Verification items for the finished model (mm, model axes). A direction names the side the tool comes from. Give positions to 0.01 mm unless a question says otherwise; leave off trailing zeros.
from build123d import *

# Parameters (mm, degrees)
BOSS_EXTRUDE1_START = -13.97
BOSS_EXTRUDE1_DEPTH = 7.62
SKETCH3_W           = 157.48
SKETCH3_H           = 157.48
CUT_EXTRUDE1_DEPTH  = 1
SKETCH3_3_R         = 1.8
BOSS_EXTRUDE2_DEPTH = 37
FILLET1_R           = 1
SKETCH11_R          = 5.1
CUT_EXTRUDE2_DEPTH  = 12.7
SKETCH10_R          = 5
BOSS_EXTRUDE3_DEPTH = 12.5
FILLET2_R           = 1


# Read off the part's stored shape, not the designer's step: Boss-Extrude1
with BuildPart() as part:
    # Sketch1 → Revolve1 (revolve)
    with BuildSketch(Plane.YZ, mode=Mode.PRIVATE) as revolve1_sk:
        Polygon((0, 0), (-152.4, 0), (-152.4, -6.35), (-150.8, -6.35), (-150.8, -13.97), (-152.4, -13.97), (-152.4, -17.97), (-88.9, -17.97), (-88.9, -23.97), (-111.6, -30.32), (0, -30.32), align=None)
    revolve(revolve1_sk.sketch.rotate(Axis((0, 0, -30.32), (0, 0, 1)), 180), axis=Axis((0, 0, -30.32), (0, 0, 1)))

    # Boss-Extrude1 outline → Boss-Extrude1 (add)
    with BuildSketch(Plane.XY.offset(BOSS_EXTRUDE1_START)):
        with BuildLine():
            Line((150.751862012, 3.81), (152.352367556, 3.81))
            ThreePointArc((152.352367556, 3.81), (149.471676733, 29.731765076), (142.213257992, 54.782745927))
            Line((142.213257992, 54.782745927), (140.734583678, 54.170258971))
            ThreePointArc((140.734583678, 54.170258971), (147.902420285, 29.41962056), (150.751862012, 3.81))
        make_face()
        with BuildLine():
            ThreePointArc((142.213257992, -54.782745926), (149.471676733, -29.731765075), (152.352367556, -3.81))
            Line((152.352367556, -3.81), (150.751862012, -3.81))
            ThreePointArc((150.751862012, -3.81), (147.902420285, -29.41962056), (140.734583678, -54.170258971))
            Line((140.734583678, -54.170258971), (142.213257992, -54.782745926))
        make_face()
        with BuildLine():
            Line((137.818535923, 61.210221009), (139.297210238, 61.822707964))
            ThreePointArc((139.297210238, 61.822707964), (126.715968915, 84.668903512), (110.423469065, 105.035315393))
            Line((110.423469065, 105.035315393), (109.291740741, 103.903587069))
            ThreePointArc((109.291740741, 103.903587069), (125.385617535, 83.77999114), (137.818535923, 61.210221009))
        make_face()
        with BuildLine():
            ThreePointArc((110.423469065, -105.035315392), (126.715968915, -84.668903512), (139.297210238, -61.822707964))
            Line((139.297210238, -61.822707964), (137.818535923, -61.210221009))
            ThreePointArc((137.818535923, -61.210221009), (125.385617535, -83.77999114), (109.291740741, -103.903587069))
            Line((109.291740741, -103.903587069), (110.423469065, -105.035315392))
        make_face()
        with BuildLine():
            Line((103.903587069, 109.291740741), (105.035315393, 110.423469065))
            ThreePointArc((105.035315393, 110.423469065), (84.668903512, 126.715968915), (61.822707964, 139.297210238))
            Line((61.822707964, 139.297210238), (61.210221009, 137.818535923))
            ThreePointArc((61.210221009, 137.818535923), (83.77999114, 125.385617535), (103.903587069, 109.291740741))
        make_face()
        with BuildLine():
            ThreePointArc((61.822707964, -139.297210238), (84.668903512, -126.715968915), (105.035315393, -110.423469065))
            Line((105.035315393, -110.423469065), (103.903587069, -109.291740741))
            ThreePointArc((103.903587069, -109.291740741), (83.77999114, -125.385617535), (61.210221009, -137.818535923))
            Line((61.210221009, -137.818535923), (61.822707964, -139.297210238))
        make_face()
        with BuildLine():
            Line((54.170258971, 140.734583678), (54.782745927, 142.213257992))
            ThreePointArc((54.782745927, 142.213257992), (29.731765076, 149.471676733), (3.81, 152.352367556))
            Line((3.81, 152.352367556), (3.81, 150.751862012))
            ThreePointArc((3.81, 150.751862012), (29.41962056, 147.902420285), (54.170258971, 140.734583678))
        make_face()
        with BuildLine():
            ThreePointArc((3.81, -152.352367556), (29.731765076, -149.471676733), (54.782745927, -142.213257992))
            Line((54.782745927, -142.213257992), (54.170258971, -140.734583678))
            ThreePointArc((54.170258971, -140.734583678), (29.41962056, -147.902420285), (3.81, -150.751862012))
            Line((3.81, -150.751862012), (3.81, -152.352367556))
        make_face()
        with BuildLine():
            Line((-3.81, 150.751862012), (-3.81, 152.352367556))
            ThreePointArc((-3.81, 152.352367556), (-29.731765076, 149.471676733), (-54.782745927, 142.213257992))
            Line((-54.782745927, 142.213257992), (-54.170258971, 140.734583678))
            ThreePointArc((-54.170258971, 140.734583678), (-29.41962056, 147.902420285), (-3.81, 150.751862012))
        make_face()
        with BuildLine():
            ThreePointArc((-54.782745926, -142.213257992), (-29.731765075, -149.471676733), (-3.81, -152.352367556))
            Line((-3.81, -152.352367556), (-3.81, -150.751862012))
            ThreePointArc((-3.81, -150.751862012), (-29.41962056, -147.902420285), (-54.170258971, -140.734583678))
            Line((-54.170258971, -140.734583678), (-54.782745926, -142.213257992))
        make_face()
        with BuildLine():
            Line((-61.210221009, 137.818535923), (-61.822707964, 139.297210238))
            ThreePointArc((-61.822707964, 139.297210238), (-84.668903512, 126.715968915), (-105.035315393, 110.423469065))
            Line((-105.035315393, 110.423469065), (-103.903587069, 109.291740741))
            ThreePointArc((-103.903587069, 109.291740741), (-83.77999114, 125.385617535), (-61.210221009, 137.818535923))
        make_face()
        with BuildLine():
            ThreePointArc((-105.035315392, -110.423469065), (-84.668903512, -126.715968915), (-61.822707964, -139.297210238))
            Line((-61.822707964, -139.297210238), (-61.210221009, -137.818535923))
            ThreePointArc((-61.210221009, -137.818535923), (-83.77999114, -125.385617535), (-103.903587069, -109.291740741))
            Line((-103.903587069, -109.291740741), (-105.035315392, -110.423469065))
        make_face()
        with BuildLine():
            Line((-109.291740741, 103.903587069), (-110.423469065, 105.035315393))
            ThreePointArc((-110.423469065, 105.035315393), (-126.715968915, 84.668903512), (-139.297210238, 61.822707964))
            Line((-139.297210238, 61.822707964), (-137.818535923, 61.210221009))
            ThreePointArc((-137.818535923, 61.210221009), (-125.385617535, 83.77999114), (-109.291740741, 103.903587069))
        make_face()
        with BuildLine():
            ThreePointArc((-139.297210238, -61.822707964), (-126.715968915, -84.668903512), (-110.423469065, -105.035315393))
            Line((-110.423469065, -105.035315393), (-109.291740741, -103.903587069))
            ThreePointArc((-109.291740741, -103.903587069), (-125.385617535, -83.77999114), (-137.818535923, -61.210221009))
            Line((-137.818535923, -61.210221009), (-139.297210238, -61.822707964))
        make_face()
        with BuildLine():
            Line((-140.734583678, 54.170258971), (-142.213257992, 54.782745926))
            ThreePointArc((-142.213257992, 54.782745926), (-149.471676733, 29.731765075), (-152.352367556, 3.81))
            Line((-152.352367556, 3.81), (-150.751862012, 3.81))
            ThreePointArc((-150.751862012, 3.81), (-147.902420285, 29.41962056), (-140.734583678, 54.170258971))
        make_face()
        with BuildLine():
            ThreePointArc((-152.352367556, -3.81), (-149.471676733, -29.731765076), (-142.213257992, -54.782745927))
            Line((-142.213257992, -54.782745927), (-140.734583678, -54.170258971))
            ThreePointArc((-140.734583678, -54.170258971), (-147.902420285, -29.41962056), (-150.751862012, -3.81))
            Line((-150.751862012, -3.81), (-152.352367556, -3.81))
        make_face()
    extrude(amount=BOSS_EXTRUDE1_DEPTH)

    # Sketch3 → Cut-Extrude1 (cut)
    with BuildSketch(Plane(origin=(0, 0, -30.32), x_dir=(1, 0, 0), z_dir=(0, 0, -1))):
        Rectangle(SKETCH3_W, SKETCH3_H)
    extrude(amount=-CUT_EXTRUDE1_DEPTH, mode=Mode.SUBTRACT)

    # Sketch3<3> → Boss-Extrude2 (add)
    with BuildSketch(Plane(origin=(0, 0, -30.32), x_dir=(1, 0, 0), z_dir=(0, 0, -1))):
        with Locations(Location((0, 0, 0), (0, 0, 180))):
            Circle(SKETCH3_3_R)
    extrude(amount=-BOSS_EXTRUDE2_DEPTH)

    # Fillet1
    fillet1_edges = [part.edges().sort_by_distance(p)[0] for p in [
        (1.8, 0, 6.68),
    ]]
    fillet(fillet1_edges, radius=FILLET1_R)

    # Split2
    split(bisect_by=Plane(origin=(0, 0, 0), x_dir=(-0.9807852804032318, -0.19509032201612173, 0), z_dir=(0.19509032201612173, -0.9807852804032318, 0)), keep=Keep.BOTTOM)

    # Split3
    split(bisect_by=Plane(origin=(0, 0, 0), x_dir=(0.1951383847238072, -0.9807757189120169, 0), z_dir=(-0.9807757189120169, -0.1951383847238072, 0)), keep=Keep.BOTTOM)

    # Sketch11 → Cut-Extrude2 (cut)
    with BuildSketch(Plane(origin=(0, 0, 0), x_dir=(0.9807852804032318, 0.19509032201612175, 0), z_dir=(0.19509032201612175, -0.9807852804032318, 0))):
        with Locations((88.9, -8.985)):
            Circle(SKETCH11_R)
        with Locations((120.65, -8.985)):
            Circle(SKETCH11_R)
        with Locations((41.041303899, -8.985)):
            Circle(SKETCH11_R)
    extrude(amount=-CUT_EXTRUDE2_DEPTH, mode=Mode.SUBTRACT)

    # Sketch10 → Boss-Extrude3 (add)
    with BuildSketch(Plane(origin=(0, 0, 0), x_dir=(0.19513838472380637, -0.980775718912017, 0), z_dir=(-0.980775718912017, -0.19513838472380637, 0))):
        with Locations((-120.65, -8.985)):
            Circle(SKETCH10_R)
        with Locations((-88.9, -8.985)):
            Circle(SKETCH10_R)
        with Locations((-41.041695232, -8.985)):
            Circle(SKETCH10_R)
    extrude(amount=BOSS_EXTRUDE3_DEPTH)

    # Fillet2
    fillet2_edges = [part.edges().sort_by_distance(p)[0] for p in [
        (-36.778834527, 120.795239272, -8.985),
        (-30.583190812, 89.655610197, -8.985),
        (-21.244198524, 42.717346933, -8.985),
    ]]
    fillet(fillet2_edges, radius=FILLET2_R)


solid = part.part
(1) Set-up check for faces 1 (the flat face through (-20.28, 37.87, -8.93)), 2 (the flat face through (59, 99, -17.97)), 3 (the cylindrical face through (0.1, 150.8, -10.2)): record each of +Z, -Z, +X, -X, +Y, -Y from which the full face is reachable in a straight line by a thin tool's end or side.
Solved:
face 1: +Z, -Z, -X, -Y
face 2: +X, +Y
face 3: +Y
(2) Scan lines: line 1 (Z direction, x = 86.5, y = 100); line 2 (Z direction, x = 20, y = 108); line 3 (Z direction, x = 25, y = 53). Record each from-to range of solid material in increasing order.
Solved:
line 1: z = -17.97 to 0
line 2: z = -30.32 to -29.83, -17.97 to 0
line 3: z = -29.32 to 0
(3) Release check for a two-part mould opening along Z. For faces 4 (the flat face through (31, 39, -29.32)), 5 (the flat face through (-35.814, 115.946, -8.929)), 6 (the flat face through (107, 107, -13.97)) record: pulls with the +Z half, pulls with the -Z half, needs draft (parallel to the pull), parting line crosses it, or undercut.
Solved:
face 4: pulls with the -Z half
face 5: needs draft
face 6: undercut
(4) Go/stop test with flat-tipped pins: pin 1 (3.5 mm diameter, centred on x = 139.5, y = 58.5, fed in from +Z); pin 2 (10 mm diameter, centred on x = 83.5, z = -19, fed in from +Y); pin 3 (3.5 mm diameter, centred on x = 107, y = 106, fed in from -Z); pin 4 (4 mm diameter, centred on y = 98.5, z = -23, fed in from -X). Record where each tip stops, or that it passes through.
Solved:
pin 1: stops at z = 0
pin 2: stops at y = 130.56
pin 3: stops at z = -17.97
pin 4: passes through
